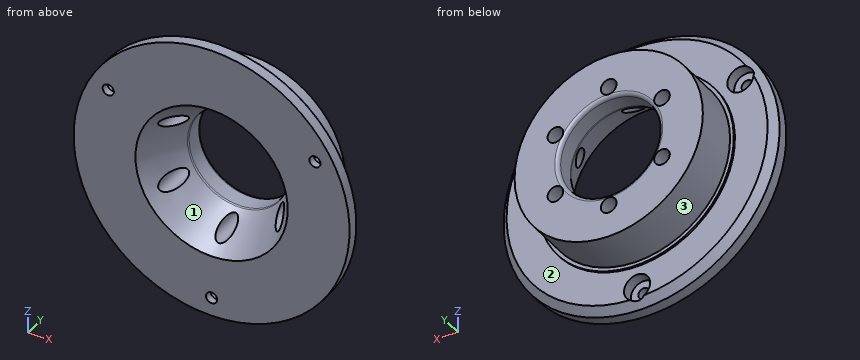
```python
from build123d import *

# Parameters (mm, degrees)
SKETCH1_R           = 25.25
SKETCH1_R_2         = 13.5
BOSS_EXTRUDE1_DEPTH = 12.5
BOSS_EXTRUDE2_START = -5
SKETCH2_R           = 37
SKETCH2_R_2         = 13.5
BOSS_EXTRUDE2_DEPTH = 5
SKETCH3_R           = 1.5000000000000004
CUT_EXTRUDE1_DEPTH  = 54.79823417176441
CUT_EXTRUDE2_START  = -3
SKETCH4_R           = 3.500000000000001
CUT_EXTRUDE2_DEPTH  = 57.79823417176441
CIRPATTERN1_COUNT   = 3
CHAMFER1_SIZE       = 12
CHAMFER1_SIZE2      = 6.928203230275528
CHAMFER2_SIZE       = 2
SKETCH5_R           = 2.100000000000002
CUT_EXTRUDE3_DEPTH  = 56.174722607367954
CIRPATTERN2_COUNT   = 6
FILLET1_R           = 1
SKETCH6_R           = 26.250000000000004
SKETCH6_R_2         = 25.25
BOSS_EXTRUDE3_DEPTH = 0.5


with BuildPart() as part:
    # Sketch1 → Boss-Extrude1 (new body)
    with BuildSketch(Plane(origin=(0, 0, 0), x_dir=(1, 0, 0), z_dir=(0, 1, 0))):
        with Locations(Location((0, 0, 0), (0, 0, 270))):
            Circle(SKETCH1_R)
        with Locations(Location((0, 0, 0), (0, 0, 270))):
            Circle(SKETCH1_R_2, mode=Mode.SUBTRACT)
    extrude(amount=BOSS_EXTRUDE1_DEPTH)

    # Sketch2 → Boss-Extrude2 (add)
    with BuildSketch(Plane(origin=(0, 0, 0), x_dir=(1, 0, 0), z_dir=(0, 1, 0)).offset(BOSS_EXTRUDE2_START)):
        with Locations(Location((0, 0, 0), (0, 0, 270))):
            Circle(SKETCH2_R)
        with Locations(Location((0, 0, 0), (0, 0, 270))):
            Circle(SKETCH2_R_2, mode=Mode.SUBTRACT)
    extrude(amount=BOSS_EXTRUDE2_DEPTH)

    # Sketch3 → Cut-Extrude1 (cut, through all)
    with BuildSketch(Plane(origin=(0, 0, 0), x_dir=(1, 0, 0), z_dir=(0, 1, 0))):
        with Locations(Location((0, 32, 0), (0, 0, 270))):
            Circle(SKETCH3_R)
    cut_extrude1 = extrude(amount=-CUT_EXTRUDE1_DEPTH, mode=Mode.SUBTRACT)

    # Sketch4 → Cut-Extrude2 (cut)
    with BuildSketch(Plane(origin=(0, 0, 0), x_dir=(1, 0, 0), z_dir=(0, 1, 0)).offset(CUT_EXTRUDE2_START)):
        with Locations(Location((0, 32, 0), (0, 0, 270))):
            Circle(SKETCH4_R)
    cut_extrude2 = extrude(amount=CUT_EXTRUDE2_DEPTH, mode=Mode.SUBTRACT)

    # CirPattern1: Cut-Extrude1, Cut-Extrude2 ×3 about axis
    cirpattern1_axis = Axis((-1.23e-15, 0, 1.87e-15), (0, 1, 0))
    add([cut_extrude1.rotate(cirpattern1_axis, i * 360 / CIRPATTERN1_COUNT) for i in range(1, CIRPATTERN1_COUNT)], mode=Mode.SUBTRACT)
    add([cut_extrude2.rotate(cirpattern1_axis, i * 360 / CIRPATTERN1_COUNT) for i in range(1, CIRPATTERN1_COUNT)], mode=Mode.SUBTRACT)

    # Chamfer1
    chamfer1_edges = [part.edges().sort_by_distance(p)[0] for p in [
        (4.13e-15, -5, -13.5),
    ]]
    chamfer1_side = [part.faces().sort_by_distance(p)[0] for p in [
        (4.13e-15, 3.75, -13.5),
    ]]
    chamfer(chamfer1_edges, length=CHAMFER1_SIZE, length2=CHAMFER1_SIZE2, reference=chamfer1_side[0])

    # Chamfer2
    # the kernel refuses this chamfer: 2 mm, written as the material it takes off along each edge
    with BuildSketch(Plane(origin=(0, 0, 0), x_dir=(-1.8e-16, 0, 1), z_dir=(-1, 0, -1.8e-16))) as chamfer2_piece_1:
        Polygon((37, -CHAMFER2_SIZE), (37 - CHAMFER2_SIZE, 0), (37, 0), align=None)
    revolve(axis=Axis((0, 0, 0), (0, 1, 0)), mode=Mode.SUBTRACT)

    # Sketch5 → Cut-Extrude3 (cut, through all)
    with BuildSketch(Plane(origin=(0, 12.5, 0), x_dir=(1, 0, 0), z_dir=(0, 1, 0))):
        with Locations(Location((-6e-17, 16.5, 0), (0, 0, 270))):
            Circle(SKETCH5_R)
    cut_extrude3 = extrude(amount=-CUT_EXTRUDE3_DEPTH, mode=Mode.SUBTRACT)

    # CirPattern2: Cut-Extrude3 ×6 about axis
    cirpattern2_axis = Axis((-1.951e-14, 0, 4.7e-16), (0, 1, 0))
    for i in range(1, CIRPATTERN2_COUNT):
        add(cut_extrude3.rotate(cirpattern2_axis, i * 360 / CIRPATTERN2_COUNT), mode=Mode.SUBTRACT)

    # Fillet1
    # the kernel refuses this fillet: 1 mm, written as the material it takes off along each edge
    with BuildSketch(Plane(origin=(0, 7, 0), x_dir=(-1.8e-16, 0, 1), z_dir=(-1, 0, -1.8e-16))) as fillet1_piece_1:
        with BuildLine():
            CenterArc((13.5 + FILLET1_R, FILLET1_R * 0.267949192431), FILLET1_R, 180, 30.000000000000057)
            Line((13.5 + FILLET1_R * 0.133974596216, -FILLET1_R * 0.232050807569), (13.5, 0))
            Line((13.5, 0), (13.5, FILLET1_R * 0.267949192431))
        make_face()
    revolve(axis=Axis((0, 7, 0), (0, 1, 0)), mode=Mode.SUBTRACT)
    with BuildSketch(Plane(origin=(0, 12.5, 0), x_dir=(-1.8e-16, 0, 1), z_dir=(-1, 0, -1.8e-16))) as fillet1_piece_2:
        with BuildLine():
            CenterArc((13.5 + FILLET1_R, -FILLET1_R), FILLET1_R, 90, 90)
            Line((13.5 + FILLET1_R, 0), (13.5, 0))
            Line((13.5, 0), (13.5, -FILLET1_R))
        make_face()
    revolve(axis=Axis((0, 12.5, 0), (0, 1, 0)), mode=Mode.SUBTRACT)

    # Sketch6 → Boss-Extrude3 (add)
    with BuildSketch(Plane(origin=(0, 0, 0), x_dir=(1, 0, 0), z_dir=(0, 1, 0))):
        with Locations(Location((0, 0, 0), (0, 0, 270))):
            Circle(SKETCH6_R)
        with Locations(Location((0, 0, 0), (0, 0, 270))):
            Circle(SKETCH6_R_2, mode=Mode.SUBTRACT)
    extrude(amount=BOSS_EXTRUDE3_DEPTH)


solid = part.part
```
For this review, take the finished solid that the model builds, in its own axes (mm). Face numbers are marked on the shaded views. Give positions to 0.01 mm unless a question says otherwise; leave off trailing zeros. Write each loop counter-clockwise with the first axis right and the second up, starting at its lowest first coordinate (ties: lowest second). Pieces come first, ordered by that corner, then holes. Notation, with made-up numbers: M 78.5,18 L 136.5,18 A34 cw 136.5,48 Z; hole C 30.25,50 d1. An arc over 180 degrees is marked long. Answer as a JSON object with one key per item and string values. Group by question number.
Item 1: Draft analysis for pull direction X (two halves, no side actions). For the marked faces 1, 2 and 3, state which applies: +X half, -X half, draft (parallel to the pull), parting line (faces both ways), or undercut.
Item 2: Consider section A-A on z = 0. Write out the cut boundary in (x, y).
Item 3: For probe 1 along X at (y, z) = (-4.3, 16); probe 2 along X at (y, z) = (6.5, 9); probe 3 along Y at (x, z) = (2.5, 31), list the stretches that pass through material, from the lowest coordinate up. Write a range as [from, to].
Item 4: For pin 1 Ø5 at (x, y) = (-23, 8.5) entering from +Z; pin 2 Ø3.5 at (x, z) = (-14.29, 8.25) entering from -Y; pin 3 Ø1.5 at (y, z) = (3, -23.5) entering from -X; pin 4 Ø5.5 at (x, z) = (0, -33) entering from +Y, all flat-tipped, find the tip position at first contact; note any pin that passes through.
Item 5: Consider section B-B on y = 9. Write out the cut boundary in (x, z), plus the area to 3 significant figures.
Check result:
{
 "1": {"face 1": "undercut", "face 2": "draft", "face 3": "parting line"},
 "2": {"outline": "M -37,-5 L -20.43,-5 L -13.63,6.77 A1 ccw -13.5,7.27 L -13.5,11.5 A1 ccw -14.5,12.5 L -25.25,12.5 L -25.25,0.5 L -26.25,0.5 L -26.25,0 L -35,0 L -37,-2 Z; M 13.5,7.27 A1 ccw 13.63,6.77 L 20.43,-5 L 37,-5 L 37,-2 L 35,0 L 26.25,0 L 26.25,0.5 L 25.25,0.5 L 25.25,12.5 L 14.5,12.5 A1 ccw 13.5,11.5 Z"},
 "3": {"probe 1": "x = [-33.36, -29.21], [-26.21, -12.04], [12.04, 26.21], [29.21, 33.36]", "probe 2": "x = [-23.59, -16.25], [-12.33, -10.45], [10.45, 12.33], [16.25, 23.59]", "probe 3": "y = [-5, 0]"},
 "4": {"pin 1": "stops at z = 14.74", "pin 2": "passes through", "pin 3": "stops at x = -10.95", "pin 4": "stops at y = 0"},
 "5": {"outline": "C 0,0 d50.5; hole C -14.29,-8.25 d4.2; hole C -14.29,8.25 d4.2; hole C 0,0 d27; hole C 0,-16.5 d4.2; hole C 0,16.5 d4.2; hole C 14.29,-8.25 d4.2; hole C 14.29,8.25 d4.2", "area": "1,350 mm^2"}
}
